```python
from build123d import *

# Parameters (mm, degrees)
SKETCH1_R           = 35
BOSS_EXTRUDE1_DEPTH = 100
CHAMFER1_SIZE       = 10
CHAMFER1_SIZE2      = 3.639702343
CHAMFER2_SIZE       = 7
CHAMFER2_SIZE2      = 5.873697418
SKETCH2_R           = 31
CUT_EXTRUDE1_DEPTH  = 5
FILLET1_R           = 10


with BuildPart() as part:
    # Sketch1 → Boss-Extrude1 (new body)
    with BuildSketch(Plane(origin=(0, 0, 0), x_dir=(1, 0, 0), z_dir=(0, 1, 0))):
        with Locations(Location((0, 0, 0), (0, 0, 270))):
            Circle(SKETCH1_R)
    extrude(amount=BOSS_EXTRUDE1_DEPTH)

    # Chamfer1
    chamfer1_edges = [part.edges().sort_by_distance(p)[0] for p in [
        (0, 100, -35),
    ]]
    chamfer1_side = [part.faces().sort_by_distance(p)[0] for p in [
        (0, 50, -35),
    ]]
    chamfer(chamfer1_edges, length=CHAMFER1_SIZE, length2=CHAMFER1_SIZE2, reference=chamfer1_side[0])

    # Chamfer2
    chamfer2_edges = [part.edges().sort_by_distance(p)[0] for p in [
        (0, 0, -35),
    ]]
    chamfer2_side = [part.faces().sort_by_distance(p)[0] for p in [
        (0, 0, 0),
    ]]
    chamfer(chamfer2_edges, length=CHAMFER2_SIZE, length2=CHAMFER2_SIZE2, reference=chamfer2_side[0])

    # Sketch2 → Cut-Extrude1 (cut)
    with BuildSketch(Plane(origin=(0, 100, 0), x_dir=(1, 0, 0), z_dir=(0, 1, 0))):
        with Locations(Location((0, 0, 0), (0, 0, 270))):
            Circle(SKETCH2_R)
    extrude(amount=-CUT_EXTRUDE1_DEPTH, mode=Mode.SUBTRACT)

    # Fillet1
    # the kernel refuses this fillet: 10 mm, written as the material it adds along each edge
    with BuildSketch(Plane(origin=(0, 95, 0), x_dir=(0, 0, 1), z_dir=(-1, 0, 0))) as fillet1_piece_1:
        with BuildLine():
            CenterArc((22.339745962, 10), FILLET1_R, 270, 60)
            Line((22.339745962, 0), (22.339745962, -0.2))
            Line((22.339745962, -0.2), (31, -0.2))
            Line((31, -0.2), (31.2, 0))
            ThreePointArc((31.2, 0), (31.2, 2.5), (31.173205081, 4.9))
            Line((31.173205081, 4.9), (31, 5))
        make_face()
    revolve(axis=Axis((0, 95, 0), (0, 1, 0)))


solid = part.part
```
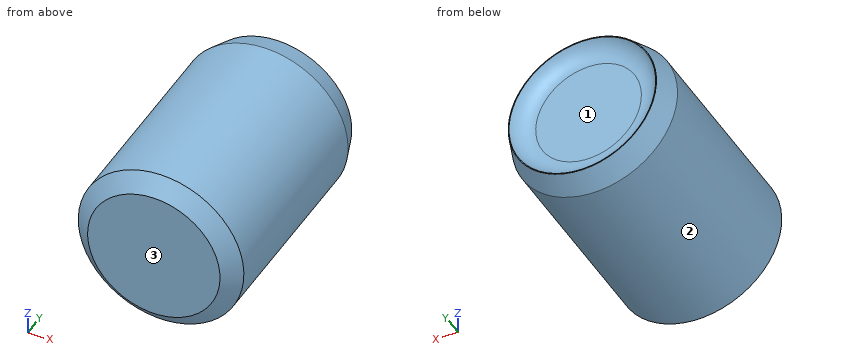
Model file for the job. Use its own axes, mm. Face numbers are marked on the shaded views. Round coordinates to 2 decimals unless told otherwise and drop trailing zeros. Write each loop counter-clockwise with the first axis right and the second up, starting at its lowest first coordinate (ties: lowest second). Pieces come first, ordered by that corner, then holes. Notation, with made-up numbers: (40.5, -13) - (49.5, -13) arc R17 ccw to (49.5, -7) - close; hole circle Ø9 at (-31.5, -36.75). An arc over 180 degrees is marked (long way). One line per item, written item: value.
(1) Wall check: probe 1 along Z at (x, y) = (21, 53); probe 2 along Y at (x, z) = (16.5, 12); probe 3 along X at (y, z) = (76.5, 0). Give the ranges that are in metal, low to high.
Values follow:
probe 1: z = -28 to 28
probe 2: y = 0 to 95
probe 3: x = -35 to 35
(2) Two-plate mould, pull along X, no slides. Class the marked faces 1, 2 and 3: pulls with the +X half, pulls with the -X half, needs draft (parallel to the pull), parting line crosses it, or undercut.
Values follow:
face 1: undercut
face 2: parting line crosses it
face 3: needs draft
(3) Drop flat-ended pins along their axis: P1, Ø1.5, axis at x = 0.5, z = 19.5, coming from the +Y side; P2, Ø1.5, axis at x = -10.5, y = 71.5, coming from the -Z side; P3, Ø6, axis at y = 16, z = 23, coming from the +X side. Give the stop position or say it passes through.
Values follow:
P1: stops at y = 95
P2: stops at z = -33.61
P3: stops at x = 28.72
(4) Cut at C-C, the plane y = 82.5. Give the cut face in (x, z).
Values follow:
outline: circle Ø70 at (0, 0)
(5) Cut at A-A, the plane z = 0. Give the cut face in (x, y).
Values follow:
outline: (-35, 5.87) - (-28, 0) - (28, 0) - (35, 5.87) - (35, 90) - (31.36, 100) - (31, 100) arc R10 cw to (22.34, 95) - (-22.34, 95) arc R10 cw to (-31, 100) - (-31.36, 100) - (-35, 90) - close
(6) Cut at B-B, the plane x = 0. Give the cut face in (y, z).
Values follow:
outline: (0, -28) - (5.87, -35) - (90, -35) - (100, -31.36) - (100, -31) arc R10 cw to (95, -22.34) - (95, 22.34) arc R10 cw to (100, 31) - (100, 31.36) - (90, 35) - (5.87, 35) - (0, 28) - close
